Design review of the part built by this model. Coordinates are the model's own, in mm. Face numbers are marked on the shaded views. A direction names the side the tool comes from. Round coordinates to 2 decimals unless told otherwise and drop trailing zeros. Loops run counter-clockwise (first coordinate to the right, second up) from the corner with the lowest first, then second, coordinate; pieces in that order, holes last. Notation, with made-up numbers: (10.25, 42.25) - (36.25, 42.25) arc R32 cw to (36.25, 81.25) - close; hole circle Ø4 at (88.5, -19). An arc over 180 degrees is marked (long way). One line per question, with ' | ' between items. Start each with the question number.
from build123d import *

# Parameters (mm, degrees)
F1_DEPTH = 22
F2_T     = -1.2
F3_DEPTH = 10
F4_SIZE  = 2
F5_SIZE  = 2


with BuildPart() as f1:
    # F0 (on Top) → F1 (new body)
    with BuildSketch(Plane.XY):
        with BuildLine():
            ThreePointArc((113, 45), (105.6776695297, 62.6776695297), (88, 70))
            Line((88, 70), (-88, 70))
            ThreePointArc((-88, 70), (-105.6776695297, 62.6776695297), (-113, 45))
            Line((-113, 45), (-113, -45))
            ThreePointArc((-113, -45), (-105.6776695297, -62.6776695297), (-88, -70))
            Line((-88, -70), (88, -70))
            ThreePointArc((88, -70), (105.6776695297, -62.6776695297), (113, -45))
            Line((113, -45), (113, 45))
        make_face()
        with BuildLine():
            ThreePointArc((106, -45), (100.7279220614, -57.7279220614), (88, -63))
            Line((88, -63), (-88, -63))
            ThreePointArc((-88, -63), (-100.7279220614, -57.7279220614), (-106, -45))
            Line((-106, -45), (-106, 45))
            ThreePointArc((-106, 45), (-100.7279220614, 57.7279220614), (-88, 63))
            Line((-88, 63), (88, 63))
            ThreePointArc((88, 63), (100.7279220614, 57.7279220614), (106, 45))
            Line((106, 45), (106, -45))
        make_face(mode=Mode.SUBTRACT)
        with BuildLine():
            Line((-88, -63), (88, -63))
            ThreePointArc((88, -63), (100.7279220614, -57.7279220614), (106, -45))
            Line((106, -45), (106, 45))
            ThreePointArc((106, 45), (100.7279220614, 57.7279220614), (88, 63))
            Line((88, 63), (-88, 63))
            ThreePointArc((-88, 63), (-100.7279220614, 57.7279220614), (-106, 45))
            Line((-106, 45), (-106, -45))
            ThreePointArc((-106, -45), (-100.7279220614, -57.7279220614), (-88, -63))
        make_face()
        with BuildLine():
            ThreePointArc((103.6, -45), (99.0308657865, -56.0308657865), (88, -60.6))
            Line((88, -60.6), (-88, -60.6))
            ThreePointArc((-88, -60.6), (-99.0308657865, -56.0308657865), (-103.6, -45))
            Line((-103.6, -45), (-103.6, 45))
            ThreePointArc((-103.6, 45), (-99.0308657865, 56.0308657865), (-88, 60.6))
            Line((-88, 60.6), (88, 60.6))
            ThreePointArc((88, 60.6), (99.0308657865, 56.0308657865), (103.6, 45))
            Line((103.6, 45), (103.6, -45))
        make_face(mode=Mode.SUBTRACT)
        with BuildLine():
            Line((-88, -60.6), (88, -60.6))
            ThreePointArc((88, -60.6), (99.0308657865, -56.0308657865), (103.6, -45))
            Line((103.6, -45), (103.6, 45))
            ThreePointArc((103.6, 45), (99.0308657865, 56.0308657865), (88, 60.6))
            Line((88, 60.6), (-88, 60.6))
            ThreePointArc((-88, 60.6), (-99.0308657865, 56.0308657865), (-103.6, 45))
            Line((-103.6, 45), (-103.6, -45))
            ThreePointArc((-103.6, -45), (-99.0308657865, -56.0308657865), (-88, -60.6))
        make_face()
    extrude(amount=F1_DEPTH)

    # F2
    f2_openings = [f1.faces().sort_by_distance(p)[0] for p in [
        (0, 0, 22),
    ]]
    offset(amount=F2_T, openings=f2_openings)

    # F0 (on Top) → F3 (join)
    with BuildSketch(Plane.XY):
        with BuildLine():
            Line((-88, -63), (88, -63))
            ThreePointArc((88, -63), (100.7279220614, -57.7279220614), (106, -45))
            Line((106, -45), (106, 45))
            ThreePointArc((106, 45), (100.7279220614, 57.7279220614), (88, 63))
            Line((88, 63), (-88, 63))
            ThreePointArc((-88, 63), (-100.7279220614, 57.7279220614), (-106, 45))
            Line((-106, 45), (-106, -45))
            ThreePointArc((-106, -45), (-100.7279220614, -57.7279220614), (-88, -63))
        make_face()
        with BuildLine():
            ThreePointArc((103.6, -45), (99.0308657865, -56.0308657865), (88, -60.6))
            Line((88, -60.6), (-88, -60.6))
            ThreePointArc((-88, -60.6), (-99.0308657865, -56.0308657865), (-103.6, -45))
            Line((-103.6, -45), (-103.6, 45))
            ThreePointArc((-103.6, 45), (-99.0308657865, 56.0308657865), (-88, 60.6))
            Line((-88, 60.6), (88, 60.6))
            ThreePointArc((88, 60.6), (99.0308657865, 56.0308657865), (103.6, 45))
            Line((103.6, 45), (103.6, -45))
        make_face(mode=Mode.SUBTRACT)
        with BuildLine():
            Line((-88, -60.6), (88, -60.6))
            ThreePointArc((88, -60.6), (99.0308657865, -56.0308657865), (103.6, -45))
            Line((103.6, -45), (103.6, 45))
            ThreePointArc((103.6, 45), (99.0308657865, 56.0308657865), (88, 60.6))
            Line((88, 60.6), (-88, 60.6))
            ThreePointArc((-88, 60.6), (-99.0308657865, 56.0308657865), (-103.6, 45))
            Line((-103.6, 45), (-103.6, -45))
            ThreePointArc((-103.6, -45), (-99.0308657865, -56.0308657865), (-88, -60.6))
        make_face()
    extrude(amount=-F3_DEPTH)

    # F4
    f4_edges = [f1.edges().sort_by_distance(p)[0] for p in [
        (0, -63, -10),
        (100.727922, -57.727922, -10),
        (106, 0, -10),
        (100.727922, 57.727922, -10),
        (0, 63, -10),
        (-100.727922, 57.727922, -10),
        (-106, 0, -10),
        (-100.727922, -57.727922, -10),
        (-113, 0, 0),
        (-105.67767, -62.67767, 0),
        (0, -70, 0),
        (-105.67767, 62.67767, 0),
        (0, 70, 0),
        (105.67767, 62.67767, 0),
        (105.67767, -62.67767, 0),
        (113, 0, 0),
    ]]
    chamfer(f4_edges, length=F4_SIZE)

    # F5
    f5_edges = [f1.edges().sort_by_distance(p)[0] for p in [
        (104.829141, 61.829141, 1.2),
        (0, 68.8, 1.2),
        (-104.829141, 61.829141, 1.2),
        (-111.8, 0, 1.2),
        (-104.829141, -61.829141, 1.2),
        (0, -68.8, 1.2),
        (104.829141, -61.829141, 1.2),
        (111.8, 0, 1.2),
    ]]
    chamfer(f5_edges, length=F5_SIZE)


solid = f1.part
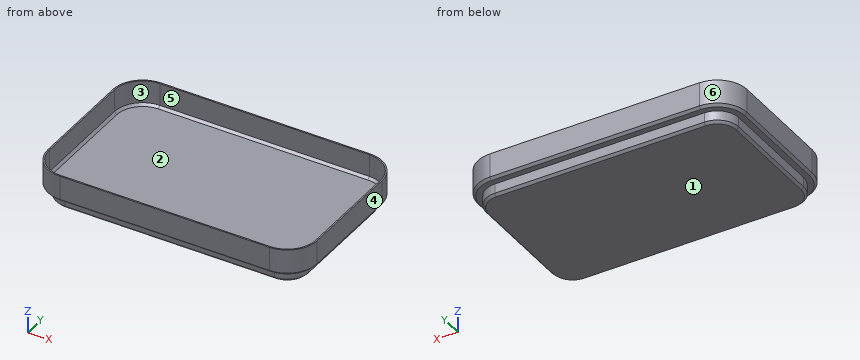
1. Clearance check with flat-ended pins moving along their axes: P1, Ø2.5, axis at x = 7.5, z = -5, coming from the +Y side; P2, Ø5, axis at y = 47, z = -3, coming from the -X side; P3, Ø4, axis at y = 12, z = -3.5, coming from the +X side. State where each tip first meets the part, or that it passes through.
2. To check wall thickness, follow line 1 along X through (y, z) = (10.5, 13); line 2 along Y through (x, z) = (-19, 15.5); line 3 along Z through (x, y) = (-16.5, -38). State the ranges of each line that lie inside material, in increasing order.
3. Take a section at D-D, the plane z = -4.5. Give the boundary of the cut face in (x, y).
4. Take a section at B-B, the plane x = 61. Give the boundary of the cut face in (y, z).
5. Machinability: for the marked faces 1 and 2, which of the approach directions +Z, -Z, +X, -X, +Y, -Y give a long, thin tool a straight path to every point of the face, cutting with its end or side? Answer none if there is none.
6. The part is to be moulded in two halves that separate along Y. For the marked faces 3, 4, 5 and 6, say which applies: pulls with the +Y half, pulls with the -Y half, needs draft (parallel to the pull), parting line crosses it, or undercut.
7. Take a section at A-A, the plane z = 6. Give the boundary of the cut face in (x, y).
8. Take a section at C-C, the plane y = -4. Give the boundary of the cut face in (x, z).
Answer list:
1) P1: stops at y = 63 | P2: stops at x = -106 | P3: stops at x = 106
2) line 1: x = -113 to -111.8, 111.8 to 113 | line 2: y = -70 to -68.8, 68.8 to 70 | line 3: z = -10 to 1.2
3) outline: (-106, -45) arc R18 ccw to (-88, -63) - (88, -63) arc R18 ccw to (106, -45) - (106, 45) arc R18 ccw to (88, 63) - (-88, 63) arc R18 ccw to (-106, 45) - close
4) outline: (-70, 2) - (-68, 0) - (-63, 0) - (-63, -8) - (-61, -10) - (61, -10) - (63, -8) - (63, 0) - (68, 0) - (70, 2) - (70, 22) - (68.8, 22) - (68.8, 3.2) - (66.8, 1.2) - (-66.8, 1.2) - (-68.8, 3.2) - (-68.8, 22) - (-70, 22) - close
5) face 1: -Z, +X, -X, +Y, -Y | face 2: +Z
6) face 3: undercut | face 4: needs draft | face 5: undercut | face 6: pulls with the +Y half
7) outline: (-113, -45) arc R25 ccw to (-88, -70) - (88, -70) arc R25 ccw to (113, -45) - (113, 45) arc R25 ccw to (88, 70) - (-88, 70) arc R25 ccw to (-113, 45) - close; hole (-111.8, -45) arc R23.8 ccw to (-88, -68.8) - (88, -68.8) arc R23.8 ccw to (111.8, -45) - (111.8, 45) arc R23.8 ccw to (88, 68.8) - (-88, 68.8) arc R23.8 ccw to (-111.8, 45) - close
8) outline: (-113, 2) - (-111, 0) - (-106, 0) - (-106, -8) - (-104, -10) - (104, -10) - (106, -8) - (106, 0) - (111, 0) - (113, 2) - (113, 22) - (111.8, 22) - (111.8, 3.2) - (109.8, 1.2) - (-109.8, 1.2) - (-111.8, 3.2) - (-111.8, 22) - (-113, 22) - close
